Autodesk Inventor part; units mm, degrees
ref_plane "YZ Plane" through (0, 0, 0) normal (1, 0, 0) x (0, 1, 0)
ref_plane "XZ Plane" through (0, 0, 0) normal (0, 1, 0) x (-1, 0, 0)
ref_plane "XY Plane" through (0, 0, 0) normal (0, 0, 1) x (1, 0, 0)
sketch "Sketch1" plane through (0, 0, 0) normal (0, 0, 1) x (1, 0, 0)
  line L0 (3.175, 0.8507) -> (3.175, -0.8507)
  line L1 (3.175, -0.8507) -> (2.3243, -2.3243)
  line L2 (2.3243, -2.3243) -> (0.8507, -3.175)
  line L3 (0.8507, -3.175) -> (-0.8507, -3.175)
  line L4 (-0.8507, -3.175) -> (-2.3243, -2.3243)
  line L5 (-2.3243, -2.3243) -> (-3.175, -0.8507)
  line L6 (-3.175, -0.8507) -> (-3.175, 0.8507)
  line L7 (-3.175, 0.8507) -> (-2.3243, 2.3243)
  line L8 (-2.3243, 2.3243) -> (-0.8507, 3.175)
  line L9 (-0.8507, 3.175) -> (0.8507, 3.175)
  line L10 (0.8507, 3.175) -> (2.3243, 2.3243)
  line L11 (2.3243, 2.3243) -> (3.175, 0.8507)
  line L12 (0, 0) -> (0, 3.175) construction
  dimension "d9" = 6.35
extrude "Extrusion1" add sketch "Sketch1" along normal mid plane 76.2
sketch "Sketch2" plane through (0, 0, 0) normal (0, 1, 0) x (-1, 0, 0)
  circle A0 centre (0, 0) radius 3.175
  dimension "diamCamSlot" = 6.35
extrude "Extrusion2" add sketch "Sketch2" along normal blind 12.7
sketch "Sketch4" plane through (0, 0, 0) normal (1, 0, 0) x (0, 1, 0)
  line L0 (12.7, -3.175) -> (12.7, 3.175)
  arc A0 (12.7, 0) -> (9.525, 3.175) centre (9.525, 0) ccw
  line L1 (9.525, 3.175) -> (12.7, 3.175)
  line L2 (3.175, 3.175) -> (12.7, 3.175)
  line L3 (12.7, 0) -> (12.7, 3.175)
  line L4 (12.7, 0) -> (9.525, 0) construction
  point P0 (0, 0)
  dimension "camRadius" = 3.175
revolve "Revolution1" cut sketch "Sketch4" angle 360 about axis through (0, 12.7, 0) along (0, -1, 0)
equation "\"d9\" = camDiam"
equation "\"diamCamSlot\" = camDiam"
equation "\"camRadius\" = 0.5 * camDiam"
equation "\"camDiam\" = 6.35"
properties part number "vexCamPost"
Read the model definition and answer for the solid it produces. Units are mm, in the model's axes. A direction names the side the tool comes from. Give positions to 0.01 mm unless a question says otherwise; leave off trailing zeros. Loops run counter-clockwise (first coordinate to the right, second up) from the corner with the lowest first, then second, coordinate; pieces in that order, holes last.
Item 1: Find the intervals of material crossed by line 1 along Y through (x, z) = (-0.5, -9) (3 decimals); line 2 along Y through (x, z) = (2.5, -8.5), in increasing order.
Item 2: The part is cut by section A-A (z = -19). Write down the section's boundary in (x, y) (3 decimals).
Item 3: Each of these flat-tipped pins is pushed along its axis until it touches: pin 1 Ø1 at (x, z) = (1, 9) entering from +Y (3 decimals); pin 2 Ø1 at (x, z) = (-2, -9.5) entering from +Y. Where does it stop, or does it pass through?
Item 4: For faces 1 (the flat face through (-2.756, 1.577, 18.783)), 2 (the cylindrical face through (-2.93, 6.09, 1.22)), 3 (the flat face through (2.744, 1.598, 18.783)), determine the directions among +Z, -Z, +X, -X, +Y, -Y from which every point of the face is accessible in a straight line to the end or side of a thin tool.
Item 5: The part is cut by section B-B (x = 0). Write down the section's boundary in (y, z) (3 decimals), and give its area (3 significant figures).
Item 6: The part is cut by section C-C (y = 4). Write down the section's boundary in (x, z) (3 decimals).
Taken from the geometry:
1. line 1: y = -3.175 to 3.175
1. line 2: y = -2.02 to 2.02
2. outline: (-3.175, -0.851) - (-2.324, -2.324) - (-0.851, -3.175) - (0.851, -3.175) - (2.324, -2.324) - (3.175, -0.851) - (3.175, 0.851) - (2.324, 2.324) - (0.851, 3.175) - (-0.851, 3.175) - (-2.324, 2.324) - (-3.175, 0.851) - close
3. pin 1: stops at y = 3.175
3. pin 2: stops at y = 2.8
4. face 1: +Z, -X, +Y
4. face 2: +Y
4. face 3: +Z, +X, +Y
5. outline: (-3.175, -38.1) - (3.175, -38.1) - (3.175, -3.175) - (9.525, -3.175) arc R3.175 ccw to (9.525, 3.175) - (3.175, 3.175) - (3.175, 38.1) - (-3.175, 38.1) - close
5. area: 540 mm2
6. outline: circle Ø6.35 at (0, 0)
